Input: part model. Units: mm. Frame: model coordinates. Face numbers are marked on the shaded views. A direction names the side the tool comes from. Round coordinates to 2 decimals unless told otherwise and drop trailing zeros. Loops run counter-clockwise (first coordinate to the right, second up) from the corner with the lowest first, then second, coordinate; pieces in that order, holes last.
(1) First-contact query: pin 1 Ø10 at (x, y) = (28.5, 7.5) entering from +Z; pin 2 Ø1 at (x, y) = (30.5, 4) entering from +Z; pin 3 Ø2 at (x, z) = (5.5, 1.5) entering from -Y. Flat tips, straight axial feed; report the tip coordinate or a pass-through.
(2) Access query for the marked faces 1, 2 and 3. Directions: +Z, -Z, +X, -X, +Y, -Y. A direction counts if a zero-diameter tool reaches every point of the face in a straight line with its end or side. Return the directions, or none.
(3) Cut plane B-B, the plane x = 8.5. Output: boundary loops of the cut face in (y, z).
(4) Cut plane A-A, the plane z = 4. Output: boundary loops of the cut face in (x, y), and give its area (3 significant figures).
(5) Draft query along Y for the marked faces 4, 5, 6 and 7. Return one class per face: released by +Y, released by -Y, zero draft, split by the parting line, or undercut.
(6) Cut plane D-D, the plane z = 7. Output: boundary loops of the cut face in (x, y).
(7) Line query: line 1 (Y direction, x = 30.5, z = 3.1); line 2 (X direction, y = 3.5, z = 3.5); line 3 (Y direction, x = 6, z = 12.75). Output: solid intervals per line, ascending.
(8) Cut plane C-C, the plane y = 30.5. Output: boundary loops of the cut face in (x, z).
from build123d import *

# Parameters (mm, degrees)
BOX002_W          = 33
BOX002_H          = 1
BOX002_DEPTH      = 10
BOX001_W          = 1
BOX001_H          = 34
BOX001_DEPTH      = 7
BOX003_W          = 33
BOX003_H          = 1
BOX003_DEPTH      = 10
BOX004_W          = 33
BOX004_H          = 1
BOX004_DEPTH      = 10
CYLINDER_R        = 1.75
CYLINDER_DEPTH    = 4.5
CYLINDER001_R     = 1.75
CYLINDER001_DEPTH = 4.5
CYLINDER003_R     = 1.75
CYLINDER003_DEPTH = 4.5
CYLINDER002_R     = 1.75
CYLINDER002_DEPTH = 4.5
BOX_W             = 33
BOX_H             = 34
BOX_DEPTH         = 4.5


with BuildPart() as body006:
    # Box002 → Box002 (join)
    with BuildSketch(Plane(origin=(0, -0.5, 4.5), x_dir=(1, 0, 0), z_dir=(0, 0, 1))):
        with Locations((16.5, 0.5)):
            Rectangle(BOX002_W, BOX002_H)
    extrude(amount=BOX002_DEPTH)


with BuildPart() as body005:
    # Box001 → Box001 (join)
    with BuildSketch(Plane(origin=(0, -0.5, 4.5), x_dir=(1, 0, 0), z_dir=(0, 0, 1))):
        with Locations((0.5, 17)):
            Rectangle(BOX001_W, BOX001_H)
    extrude(amount=BOX001_DEPTH)


with BuildPart() as body007:
    # Box003 → Box003 (join)
    with BuildSketch(Plane(origin=(0, 33.5, 4.5), x_dir=(1, 0, 0), z_dir=(0, 0, 1))):
        with Locations((16.5, 0.5)):
            Rectangle(BOX003_W, BOX003_H)
    extrude(amount=BOX003_DEPTH)


with BuildPart() as body008:
    # Box004 → Box004 (join)
    with BuildSketch(Plane(origin=(0, -0.5, 4.5), x_dir=(1, 0, 0), z_dir=(0, 0, 1))):
        with Locations((16.5, 0.5)):
            Rectangle(BOX004_W, BOX004_H)
    extrude(amount=BOX004_DEPTH)


with BuildPart() as hole3:
    # Cylinder → Cylinder (join)
    with BuildSketch(Plane(origin=(3.5, 3.5, 1), x_dir=(1, 0, 0), z_dir=(0, 0, 1))):
        Circle(CYLINDER_R)
    extrude(amount=CYLINDER_DEPTH)


with BuildPart() as hole1:
    # Cylinder001 → Cylinder001 (join)
    with BuildSketch(Plane(origin=(3.5, 30.5, 1), x_dir=(1, 0, 0), z_dir=(0, 0, 1))):
        Circle(CYLINDER001_R)
    extrude(amount=CYLINDER001_DEPTH)


with BuildPart() as hole2:
    # Cylinder003 → Cylinder003 (join)
    with BuildSketch(Plane(origin=(30.5, 30.5, 1), x_dir=(1, 0, 0), z_dir=(0, 0, 1))):
        Circle(CYLINDER003_R)
    extrude(amount=CYLINDER003_DEPTH)


with BuildPart() as hole4:
    # Cylinder002 → Cylinder002 (join)
    with BuildSketch(Plane(origin=(30.5, 3.5, 1), x_dir=(1, 0, 0), z_dir=(0, 0, 1))):
        Circle(CYLINDER002_R)
    extrude(amount=CYLINDER002_DEPTH)


with BuildPart() as base:
    # Box → Box (join)
    with BuildSketch(Plane.XY):
        with Locations((16.5, 17)):
            Rectangle(BOX_W, BOX_H)
    extrude(amount=BOX_DEPTH)

    # Boolean: union Body006, Body005, Body007, Body008
    add(body006.part)
    add(body005.part)
    add(body007.part)
    add(body008.part)

    # Boolean001: cut hole3, hole1, hole2, hole4
    add(hole3.part, mode=Mode.SUBTRACT)
    add(hole1.part, mode=Mode.SUBTRACT)
    add(hole2.part, mode=Mode.SUBTRACT)
    add(hole4.part, mode=Mode.SUBTRACT)


solid = base.part
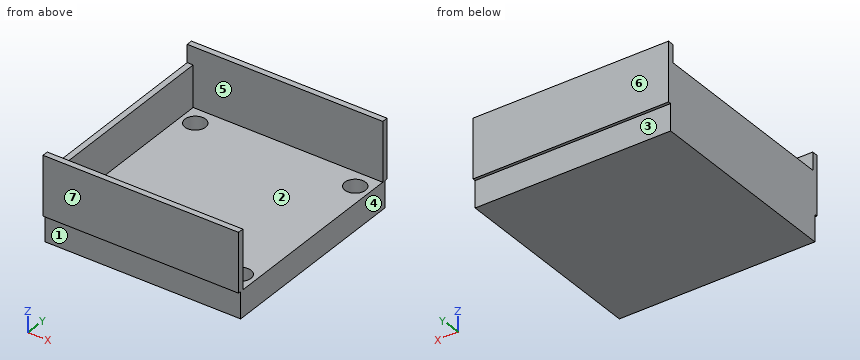
Reported:
1. pin 1: stops at z = 4.5
1. pin 2: stops at z = 1
1. pin 3: stops at y = 0
2. face 1: -Z, +X, -X, -Y
2. face 2: +Z, +X
2. face 3: -Z, +X, -X, +Y
3. outline: (-0.5, 4.5) - (0, 4.5) - (0, 0) - (34, 0) - (34, 4.5) - (34.5, 4.5) - (34.5, 14.5) - (33.5, 14.5) - (33.5, 4.5) - (0.5, 4.5) - (0.5, 14.5) - (-0.5, 14.5) - close
4. outline: (0, 0) - (33, 0) - (33, 34) - (0, 34) - close; hole circle Ø3.5 at (3.5, 3.5); hole circle Ø3.5 at (3.5, 30.5); hole circle Ø3.5 at (30.5, 3.5); hole circle Ø3.5 at (30.5, 30.5)
4. area: 1,080 mm2
5. face 4: zero draft
5. face 5: undercut
5. face 6: released by +Y
5. face 7: released by -Y
6. outline: (0, -0.5) - (33, -0.5) - (33, 0.5) - (1, 0.5) - (1, 33.5) - (33, 33.5) - (33, 34.5) - (0, 34.5) - close
7. line 1: y = 0 to 1.75, 5.25 to 28.75, 32.25 to 34
7. line 2: x = 0 to 1.75, 5.25 to 28.75, 32.25 to 33
7. line 3: y = -0.5 to 0.5, 33.5 to 34.5
8. outline: (0, 0) - (33, 0) - (33, 4.5) - (32.25, 4.5) - (32.25, 1) - (28.75, 1) - (28.75, 4.5) - (5.25, 4.5) - (5.25, 1) - (1.75, 1) - (1.75, 4.5) - (1, 4.5) - (1, 11.5) - (0, 11.5) - close
